Work out the finished part from the listing and answer in its coordinate system (mm). Face numbers are marked on the shaded views. A direction names the side the tool comes from. Round coordinates to 2 decimals unless told otherwise and drop trailing zeros. Write each loop counter-clockwise with the first axis right and the second up, starting at its lowest first coordinate (ties: lowest second). Pieces come first, ordered by that corner, then holes.
1. Find section B-B (x = 49.5). Write down the section's boundary in (y, z).
2. Find section A-A (y = -50). Write down the section's boundary in (x, z), and give its area (3 significant figures).
3. A tool of negligible diameter and unlimited length cuts with its end or side. For the marked faces 4 and 5, from which of +Z, -Z, +X, -X, +Y, -Y can it reach the whole face along a straight path? Write none if from no direction.
4. Straight lines are drawn through the part: probe 1 along Y at (x, z) = (-97, 62.1); probe 2 along X at (y, z) = (-36, 59); probe 3 along X at (y, z) = (-6, 61). For each, find the intervals that lie inside material, in ascending order.
5. Flat-ended cylindrical pins translate along their axes: pin 1 Ø8 at (x, y) = (-88.5, 8) entering from +Z; pin 2 Ø2.5 at (x, z) = (-84.5, 70) entering from -Y; pin 3 Ø12 at (x, y) = (21, -11) entering from +Z; pin 4 Ø0.6 at (x, y) = (89.5, -64) entering from -Z. Find the tip coordinate at first contact, or state that the pin passes through.
6. Determine the mould class of the marked faces 1, 2 and 3 for opening direction X: pulls with the +X half, pulls with the -X half, needs draft (parallel to the pull), parting line crosses it, or undercut.
```python
from build123d import *

# Parameters (mm, degrees)
SKETCH1_W                           = 240
SKETCH1_H                           = 138
FLOOR_2_DEPTH                       = 3
SKETCH2_W                           = 240
SKETCH2_H                           = 138
SKETCH2_W_2                         = 232
SKETCH2_H_2                         = 128
WALLS_DEPTH                         = 38
SKETCH3_R                           = 4.5
INSERT_COLUMNS_DEPTH                = 38
SKETCH4_R                           = 3
BOARD_STANDOFFS_DEPTH               = 3
SKETCH5_R                           = 1.1
STANDOFF_PILOTS_DEPTH               = 5
SKETCH6_W                           = 28
SKETCH6_H                           = 55.5
MOTOR_FLOOR_WINDOWS_DEPTH           = 4.5
MOTOR_POCKET_L_DEPTH                = 3
MOTOR_POCKET_R_DEPTH                = 3
MOTOR_SHAFT_AND_M3_HOLES_DEPTH      = 170.602476397
MOTOR_SHAFT_AND_M3_HOLES_DEPTH_BACK = 170.602476397
SKETCH9_R                           = 4
SKETCH9_R_2                         = 1.7
SKETCH10_R                          = 2
M3_INSERT_BORES_DEPTH               = 8
SKETCH11_R                          = 1.7
CRADLE_M3_HOLES_DEPTH               = 5
SKETCH12_W                          = 14
SKETCH12_H                          = 16
USB_GROMMET_DEPTH                   = 6
SKETCH13_W                          = 24
SKETCH13_H                          = 8
VENT_SLOTS_DEPTH                    = 6


with BuildPart() as part:
    # Sketch1 → Floor 2 (new body)
    with BuildSketch(Plane.XY.offset(57)):
        Rectangle(SKETCH1_W, SKETCH1_H)
    extrude(amount=FLOOR_2_DEPTH)

    # Sketch2 → Walls (add)
    with BuildSketch(Plane.XY.offset(60)):
        Rectangle(SKETCH2_W, SKETCH2_H)
        Rectangle(SKETCH2_W_2, SKETCH2_H_2, mode=Mode.SUBTRACT)
    extrude(amount=WALLS_DEPTH)

    # Sketch3 → Insert_columns (add)
    with BuildSketch(Plane.XY.offset(60)):
        with Locations((-112, 63)):
            Circle(SKETCH3_R)
        with Locations((-112, -63)):
            Circle(SKETCH3_R)
        with Locations((112, 63)):
            Circle(SKETCH3_R)
        with Locations((112, -63)):
            Circle(SKETCH3_R)
    extrude(amount=INSERT_COLUMNS_DEPTH)

    # Sketch4 → Board_standoffs (add)
    with BuildSketch(Plane.XY.offset(60)):
        with Locations((1.5, -17.5)):
            Circle(SKETCH4_R)
        with Locations((1.5, -58.5)):
            Circle(SKETCH4_R)
        with Locations((-57.5, -17.5)):
            Circle(SKETCH4_R)
        with Locations((-57.5, -58.5)):
            Circle(SKETCH4_R)
        with Locations((56, -25.5)):
            Circle(SKETCH4_R)
        with Locations((56, -58.5)):
            Circle(SKETCH4_R)
        with Locations((18, -25.5)):
            Circle(SKETCH4_R)
        with Locations((18, -58.5)):
            Circle(SKETCH4_R)
        with Locations((56, 15.5)):
            Circle(SKETCH4_R)
        with Locations((56, -17.5)):
            Circle(SKETCH4_R)
        with Locations((18, 15.5)):
            Circle(SKETCH4_R)
        with Locations((18, -17.5)):
            Circle(SKETCH4_R)
        with Locations((-2.4, 12.2)):
            Circle(SKETCH4_R)
        with Locations((-2.4, -6.2)):
            Circle(SKETCH4_R)
        with Locations((-57.6, 12.2)):
            Circle(SKETCH4_R)
        with Locations((-57.6, -6.2)):
            Circle(SKETCH4_R)
        with Locations((-107, 47.5)):
            Circle(SKETCH4_R)
        with Locations((-97, 47.5)):
            Circle(SKETCH4_R)
        with Locations((-107, 32.5)):
            Circle(SKETCH4_R)
        with Locations((-97, 32.5)):
            Circle(SKETCH4_R)
    extrude(amount=BOARD_STANDOFFS_DEPTH)

    # Sketch5 → Standoff_pilots (cut)
    with BuildSketch(Plane.XY.offset(59)):
        with Locations((1.5, -17.5)):
            Circle(SKETCH5_R)
        with Locations((1.5, -58.5)):
            Circle(SKETCH5_R)
        with Locations((-57.5, -17.5)):
            Circle(SKETCH5_R)
        with Locations((-57.5, -58.5)):
            Circle(SKETCH5_R)
        with Locations((56, -25.5)):
            Circle(SKETCH5_R)
        with Locations((56, -58.5)):
            Circle(SKETCH5_R)
        with Locations((18, -25.5)):
            Circle(SKETCH5_R)
        with Locations((18, -58.5)):
            Circle(SKETCH5_R)
        with Locations((56, 15.5)):
            Circle(SKETCH5_R)
        with Locations((56, -17.5)):
            Circle(SKETCH5_R)
        with Locations((18, 15.5)):
            Circle(SKETCH5_R)
        with Locations((18, -17.5)):
            Circle(SKETCH5_R)
        with Locations((-2.4, 12.2)):
            Circle(SKETCH5_R)
        with Locations((-2.4, -6.2)):
            Circle(SKETCH5_R)
        with Locations((-57.6, 12.2)):
            Circle(SKETCH5_R)
        with Locations((-57.6, -6.2)):
            Circle(SKETCH5_R)
        with Locations((-107, 47.5)):
            Circle(SKETCH5_R)
        with Locations((-97, 47.5)):
            Circle(SKETCH5_R)
        with Locations((-107, 32.5)):
            Circle(SKETCH5_R)
        with Locations((-97, 32.5)):
            Circle(SKETCH5_R)
    extrude(amount=STANDOFF_PILOTS_DEPTH, mode=Mode.SUBTRACT)

    # Sketch6 → Motor_floor_windows (cut)
    with BuildSketch(Plane.XY.offset(56)):
        with Locations((76, 36.75)):
            Rectangle(SKETCH6_W, SKETCH6_H)
        with Locations((76, -36.75)):
            Rectangle(SKETCH6_W, SKETCH6_H)
        with Locations((-76, 36.75)):
            Rectangle(SKETCH6_W, SKETCH6_H)
        with Locations((-76, -36.75)):
            Rectangle(SKETCH6_W, SKETCH6_H)
    extrude(amount=MOTOR_FLOOR_WINDOWS_DEPTH, mode=Mode.SUBTRACT)

    # Sketch7 → Motor_pocket_L (cut)
    with BuildSketch(Plane(origin=(0, 64, 0), x_dir=(1, 0, 0), z_dir=(0, 1, 0))):
        with BuildLine():
            Line((89, -70), (89, -52))
            Line((89, -52), (63, -52))
            Line((63, -52), (63, -70))
            ThreePointArc((63, -70), (76, -83), (89, -70))
        make_face()
        with BuildLine():
            Line((-63, -70), (-63, -52))
            Line((-63, -52), (-89, -52))
            Line((-89, -52), (-89, -70))
            ThreePointArc((-89, -70), (-76, -83), (-63, -70))
        make_face()
    extrude(amount=MOTOR_POCKET_L_DEPTH, mode=Mode.SUBTRACT)

    # Sketch8 → Motor_pocket_R (cut)
    with BuildSketch(Plane(origin=(0, -67, 0), x_dir=(1, 0, 0), z_dir=(0, 1, 0))):
        with BuildLine():
            Line((89, -70), (89, -52))
            Line((89, -52), (63, -52))
            Line((63, -52), (63, -70))
            ThreePointArc((63, -70), (76, -83), (89, -70))
        make_face()
        with BuildLine():
            Line((-63, -70), (-63, -52))
            Line((-63, -52), (-89, -52))
            Line((-89, -52), (-89, -70))
            ThreePointArc((-89, -70), (-76, -83), (-63, -70))
        make_face()
    extrude(amount=MOTOR_POCKET_R_DEPTH, mode=Mode.SUBTRACT)

    # Sketch9 → Motor_shaft_and_M3_holes (cut, two sides: drawn at the far end of the back side and taken through both)
    with BuildSketch(Plane(origin=(0, 0, 0), x_dir=(1, 0, 0), z_dir=(0, 1, 0)).offset(-MOTOR_SHAFT_AND_M3_HOLES_DEPTH_BACK)):
        with Locations(Location((76, -70, 0), (0, 0, 270))):
            Circle(SKETCH9_R)
        with Locations(Location((67.5, -70, 0), (0, 0, 270))):
            Circle(SKETCH9_R_2)
        with Locations(Location((84.5, -70, 0), (0, 0, 270))):
            Circle(SKETCH9_R_2)
        with Locations(Location((-76, -70, 0), (0, 0, 270))):
            Circle(SKETCH9_R)
        with Locations(Location((-84.5, -70, 0), (0, 0, 270))):
            Circle(SKETCH9_R_2)
        with Locations(Location((-67.5, -70, 0), (0, 0, 270))):
            Circle(SKETCH9_R_2)
    extrude(amount=MOTOR_SHAFT_AND_M3_HOLES_DEPTH + MOTOR_SHAFT_AND_M3_HOLES_DEPTH_BACK, mode=Mode.SUBTRACT)

    # Sketch10 → M3_insert_bores (cut)
    with BuildSketch(Plane.XY.offset(98)):
        with Locations((-112, 63)):
            Circle(SKETCH10_R)
        with Locations((-112, -63)):
            Circle(SKETCH10_R)
        with Locations((112, 63)):
            Circle(SKETCH10_R)
        with Locations((112, -63)):
            Circle(SKETCH10_R)
    extrude(amount=-M3_INSERT_BORES_DEPTH, mode=Mode.SUBTRACT)

    # Sketch11 → Cradle_M3_holes (cut)
    with BuildSketch(Plane.XY.offset(56)):
        with Locations((61, 42)):
            Circle(SKETCH11_R)
        with Locations((-61, 42)):
            Circle(SKETCH11_R)
    extrude(amount=CRADLE_M3_HOLES_DEPTH, mode=Mode.SUBTRACT)

    # Sketch12 → USB_grommet (cut)
    with BuildSketch(Plane(origin=(-121, 0, 0), x_dir=(0, 0, -1), z_dir=(1, 0, 0))):
        with Locations((-89, -30)):
            Rectangle(SKETCH12_W, SKETCH12_H)
    extrude(amount=USB_GROMMET_DEPTH, mode=Mode.SUBTRACT)

    # Sketch13 → Vent_slots (cut)
    with BuildSketch(Plane(origin=(115, 0, 0), x_dir=(0, 0, -1), z_dir=(1, 0, 0))):
        with Locations((-78, -50)):
            Rectangle(SKETCH13_W, SKETCH13_H)
        with Locations((-78, -25)):
            Rectangle(SKETCH13_W, SKETCH13_H)
        with Locations((-78, 0)):
            Rectangle(SKETCH13_W, SKETCH13_H)
        with Locations((-78, 25)):
            Rectangle(SKETCH13_W, SKETCH13_H)
        with Locations((-78, 50)):
            Rectangle(SKETCH13_W, SKETCH13_H)
    extrude(amount=VENT_SLOTS_DEPTH, mode=Mode.SUBTRACT)


solid = part.part
```
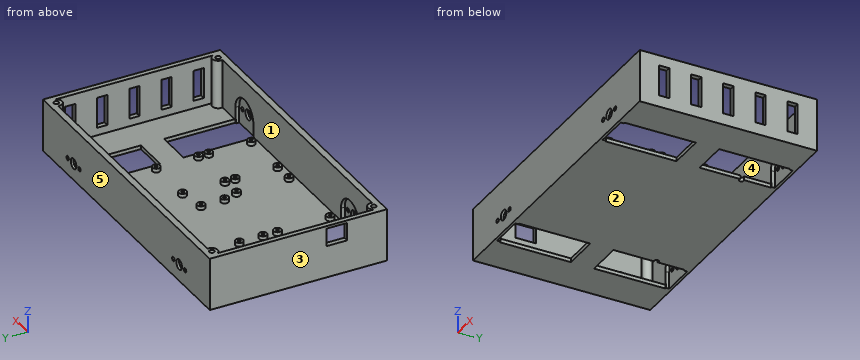
Worked answers:
1. outline: (-69, 57) - (69, 57) - (69, 98) - (64, 98) - (64, 60) - (-64, 60) - (-64, 98) - (-69, 98) - close
2. outline: (-120, 57) - (-90, 57) - (-90, 60) - (-116, 60) - (-116, 98) - (-120, 98) - close; (-62, 57) - (62, 57) - (62, 60) - (-62, 60) - close; (90, 57) - (120, 57) - (120, 66) - (116, 66) - (116, 60) - (90, 60) - close; (116, 90) - (120, 90) - (120, 98) - (116, 98) - close
2. area: 760 mm2
3. face 4: +Z
3. face 5: +Z, -Z, +X, -X, +Y
4. probe 1: y = -69 to -64, 29.5 to 31.4, 33.6 to 35.5, 44.5 to 46.4, 48.6 to 50.5, 64 to 69
4. probe 2: x = -120 to -90, -62 to 62, 90 to 120
4. probe 3: x = -120 to -116, -60.59 to -58.68, -56.52 to -54.61, -5.39 to -3.48, -1.32 to 0.59, 116 to 120
5. pin 1: stops at z = 60
5. pin 2: passes through
5. pin 3: stops at z = 63
5. pin 4: stops at z = 60.5
6. face 1: undercut
6. face 2: needs draft
6. face 3: pulls with the -X half
